Autodesk Fusion 360 part; units mm, degrees
sketch "Esboço1" plane through (0, 0, 0) normal (0, 0, 1) x (1, 0, 0)
  line L0 (0, 0) -> (120, 0)
  line L1 (120, 0) -> (120, 35)
  line L2 (120, 35) -> (0, 35)
  line L3 (0, 35) -> (0, 0)
  dimension "d1" = 120
  dimension "d2" = 35
extrude "Extrusão1" add sketch "Esboço1" along normal blind 4
sketch "Esboço2" plane through (0, 0, 4) normal (0, 0, 1) x (-1, 0, 0)
  line L0 (0, -35) -> (0, 0)
  line L1 (0, 0) -> (-120, 0)
  line L2 (-120, 0) -> (-120, -35)
  line L3 (-120, -35) -> (0, -35)
  line L4 (-10, -30) -> (-110, -30)
  line L5 (-110, -30) -> (-110, -5)
  line L6 (-110, -5) -> (-10, -5)
  line L7 (-10, -5) -> (-10, -30)
  point P0 (-5, -30)
  point P1 (-5, -5)
  point P2 (-115, -5)
  point P3 (-115, -30)
sketch "Esboço8" plane through (0, 0, 4) normal (0, 0, 1) x (1, 0, 0)
  circle A0 centre (5, 30) radius 2
  circle A1 centre (5, 5) radius 2
  circle A2 centre (115, 30) radius 2
  circle A3 centre (115, 5) radius 2
  dimension "d18" = 4
  dimension "d19" = 4
  dimension "d20" = 4
  dimension "d21" = 4
extrude "Extrusão7" cut sketch "Esboço8" against normal blind 20
extrude "Extrusão10" add sketch "Esboço2" along normal blind 3 contours L4 L5 L6 L7
sketch "Esboço10" plane through (0, 0, 7) normal (0, 0, 1) x (-1, 0, 0)
  line L0 (-10, -5) -> (-110, -5)
  line L1 (-110, -5) -> (-110, -30)
  line L2 (-110, -30) -> (-10, -30)
  line L3 (-10, -30) -> (-10, -5)
  line L4 (-110, -30) -> (-110, -21.55)
  line L5 (-110, -5) -> (-110, -13.45)
  line L6 (-110, -21.55) -> (-35.05, -21.55)
  line L7 (-110, -13.45) -> (-35.05, -13.45)
  line L8 (-35.05, -21.55) -> (-35.05, -13.45)
  dimension "d35" = 8.45
  dimension "d36" = 8.45
  dimension "d37" = 74.95
  dimension "d38" = 74.95
extrude "Extrusão11" add sketch "Esboço10" along normal blind 2.2 contours L1 L6 L7 L8
Design review of the part built by this model. Coordinates are the model's own, in mm. A direction names the side the tool comes from. Coordinates: 2 decimals unless noted, no trailing zeros. Order: outer loops, then holes, each group sorted by start corner. A loop starts at its lowest first (then second) coordinate and runs counter-clockwise, first axis right, second up. Notation, with made-up numbers: (-7.5, 10.5) -> (14.5, 10.5) arc R23 ccw to (14.5, 28.5) -> close; hole circle Ø2 at (-26.75, -40). An arc over 180 degrees is marked (long way). Use one line per item in the form item = value. Start each with the question number.
(1) For faces 5 (the flat face through (10, 17, 5)), 6 (the flat face through (73, 21.55, 8)), 7 (the flat face through (61, 5, 5)), list the 3-axis set-ups (+Z, -Z, +X, -X, +Y, -Y) from which the entire face can be reached by the end or side of a thin tool; tool diameter is ignored.
(2) Add section B-B on y = 25.5. State the section outline as (x, z) points, plus the area to 3 significant figures.
(3) Insertion check: pin 1 (10 mm diameter, centred on x = 105.5, y = 3.5, fed in from -Z); pin 2 (2.5 mm diameter, centred on x = 115, y = 5, fed in from +Z); pin 3 (2.5 mm diameter, centred on x = 76.5, z = 7.5, fed in from -Y); pin 4 (5 mm diameter, centred on x = 5, y = 5, fed in from +Z). Each pin has a flat end and moves straight along its axis. Give the tip position at first contact, or say it passes through.
(4) Add section D-D on y = 17.5. State the section outline as (x, z) points, plus the area to 3 significant figures.
(5) The part is to be moulded in two halves that separate along X. For faces 1 (the flat face through (59, 2, 4)), 2 (the flat face through (110, 18, 6)), 3 (the flat face through (35.05, 18, 8)), 4 (the cylindrical face through (3, 5, 2)), say which applies: +X half, -X half, draft (parallel to the pull), parting line (faces both ways), or undercut.
(6) Add section A-A on x = 5. State the section outline as (y, z) points, plus the area to 3 significant figures.
(7) For probe 1 along Y at (x, z) = (5, 3.05); probe 2 along X at (y, z) = (16, 8); probe 3 along Z at (x, y) = (111, 30), list the stretches that pass through material, from the lowest coordinate up.
(8) Add section C-C on x = 86.5. State the section outline as (y, z) points, plus the area to 3 significant figures.
Answer block:
q1.face_5 = +Z, -X, +Y, -Y
q1.face_6 = +Z, +X, -X, +Y
q1.face_7 = +Z, +X, -X, -Y
q2.outline = (0, 0) -> (120, 0) -> (120, 4) -> (110, 4) -> (110, 7) -> (10, 7) -> (10, 4) -> (0, 4) -> close
q2.area = 780 mm²
q3.pin_1 = 0
q3.pin_2 = through
q3.pin_3 = 5
q3.pin_4 = 4
q4.outline = (0, 0) -> (120, 0) -> (120, 4) -> (110, 4) -> (110, 9.2) -> (35.05, 9.2) -> (35.05, 7) -> (10, 7) -> (10, 4) -> (0, 4) -> close
q4.area = 945 mm²
q5.face_1 = draft
q5.face_2 = +X half
q5.face_3 = -X half
q5.face_4 = undercut
q6.outline = (0, 0) -> (3, 0) -> (3, 4) -> (0, 4) -> close; (7, 0) -> (28, 0) -> (28, 4) -> (7, 4) -> close; (32, 0) -> (35, 0) -> (35, 4) -> (32, 4) -> close
q6.area = 108 mm²
q7.probe_1 = 0 to 3, 7 to 28, 32 to 35
q7.probe_2 = 35.05 to 110
q7.probe_3 = 0 to 4
q8.outline = (0, 0) -> (35, 0) -> (35, 4) -> (30, 4) -> (30, 7) -> (21.55, 7) -> (21.55, 9.2) -> (13.45, 9.2) -> (13.45, 7) -> (5, 7) -> (5, 4) -> (0, 4) -> close
q8.area = 233 mm²
